CAD build for the part. Positions are in the model's coordinates, mm. A direction names the side the tool comes from. Coordinates: 2 decimals unless noted, no trailing zeros. Write each loop counter-clockwise with the first axis right and the second up, starting at its lowest first coordinate (ties: lowest second). Pieces come first, ordered by that corner, then holes.
Autodesk Inventor part; units mm, degrees
ref_plane "YZ Plane" through (0, 0, 0) normal (1, 0, 0) x (0, 1, 0)
ref_plane "XZ Plane" through (0, 0, 0) normal (0, 1, 0) x (-1, 0, 0)
ref_plane "XY Plane" through (0, 0, 0) normal (0, 0, 1) x (1, 0, 0)
sketch "スケッチ1" plane through (0, 0, 0) normal (0, 1, 0) x (-1, 0, 0)
  circle A0 centre (0, 0) radius 5
  dimension "d0" = 10
extrude "押し出し1" add sketch "スケッチ1" along normal blind 27.8
sketch "スケッチ2" plane through (0, 27.8, 0) normal (0, 1, 0) x (1, 0, 0)
  circle A0 centre (0, 0) radius 4
  dimension "d3" = 8
extrude "押し出し2" add sketch "スケッチ2" along normal blind 19
sketch "スケッチ3" plane through (0, 46.8, 0) normal (0, 1, 0) x (1, 0, 0)
  circle A0 centre (0, 0) radius 3
  dimension "d6" = 6
extrude "押し出し3" add sketch "スケッチ3" along normal blind 25
sketch "スケッチ4" plane through (0, 0, 0) normal (0, -1, 0) x (1, 0, 0)
  circle A0 centre (0, 0) radius 4
  circle A1 centre (0, 0) radius 4
  dimension "d9" = 8
extrude "押し出し4" add sketch "スケッチ4" along normal blind 32
sketch "スケッチ5" plane through (0, -32, 0) normal (0, -1, 0) x (1, 0, 0)
  circle A0 centre (0, 0) radius 4
  circle A1 centre (0, 0) radius 3
  dimension "d12" = 6
extrude "押し出し5" add sketch "スケッチ5" along normal blind 15 contours A1
properties part number "shoulder1_shaft2"
Item 1: Flat gauge pins, fed straight in: pin 1 Ø1.5 at (x, z) = (-4, -3) entering from +Y; pin 2 Ø3 at (x, z) = (4, 3) entering from -Y; pin 3 Ø4 at (x, y) = (0.5, -31) entering from +Z. Where does each tip first touch, or does it go through?
Item 2: Saw through at C-C, the plane y = 30.5. Write the cut outline in (x, z), and give its area (3 significant figures).
Item 3: Saw through at B-B, the plane x = 0. Write the cut outline in (y, z).
Item 4: Wall check: line 1 along Y through (x, z) = (-2, -3); line 2 along Y through (x, z) = (-3.75, 1.75); line 3 along X through (y, z) = (15, 4). Give the ranges that are in metal, low to high.
Item 5: Saw through at A-A, the plane z = 0. Write the cut outline in (x, y), and give its area (3 significant figures).
Item 6: Two-plate mould, pull along X, no slides. Class faces 4 (the cylindrical face through (-0.867, 37.167, -3.905)), 5 (the flat face through (1, 46.8, -3)): +X half, -X half, draft (parallel to the pull), parting line (faces both ways), or undercut.
Item 7: Which spindle directions (+Z, -Z, +X, -X, +Y, -Y) get a long thin tool onto all of the face, cutting with end or side? Do faces 1 (the cylindrical face through (-3, -39, 0)), 2 (the cylindrical face through (1.08, 13.71, 4.88)), 3 (the cylindrical face through (-3, 59, 0)). Say none if no direction does.
Working result:
1. pin 1: stops at y = 27.8
1. pin 2: stops at y = -32
1. pin 3: stops at z = 4
2. outline: circle Ø8 at (0, 0)
2. area: 50.3 mm2
3. outline: (-47, -3) - (-32, -3) - (-32, -4) - (0, -4) - (0, -5) - (27.8, -5) - (27.8, -4) - (46.8, -4) - (46.8, -3) - (71.8, -3) - (71.8, 3) - (46.8, 3) - (46.8, 4) - (27.8, 4) - (27.8, 5) - (0, 5) - (0, 4) - (-32, 4) - (-32, 3) - (-47, 3) - close
4. line 1: y = -32 to 46.8
4. line 2: y = 0 to 27.8
4. line 3: x = -3 to 3
5. outline: (-5, 0) - (-4, 0) - (-4, -32) - (-3, -32) - (-3, -47) - (3, -47) - (3, -32) - (4, -32) - (4, 0) - (5, 0) - (5, 27.8) - (4, 27.8) - (4, 46.8) - (3, 46.8) - (3, 71.8) - (-3, 71.8) - (-3, 46.8) - (-4, 46.8) - (-4, 27.8) - (-5, 27.8) - close
5. area: 926 mm2
6. face 4: parting line
6. face 5: draft
7. face 1: -Y
7. face 2: +Y, -Y
7. face 3: +Y
